Read the model definition and answer for the solid it produces. Units are mm, in the model's axes. A direction names the side the tool comes from. Give positions to 0.01 mm unless a question says otherwise; leave off trailing zeros. Write each loop counter-clockwise with the first axis right and the second up, starting at its lowest first coordinate (ties: lowest second). Pieces come first, ordered by that corner, then holes.
Autodesk Inventor part; units mm, degrees
ref_plane "YZ Plane" through (0, 0, 0) normal (1, 0, 0) x (0, 1, 0)
ref_plane "XZ Plane" through (0, 0, 0) normal (0, 1, 0) x (-1, 0, 0)
ref_plane "XY Plane" through (0, 0, 0) normal (0, 0, 1) x (1, 0, 0)
sketch "Sketch1" plane through (0, 0, 0) normal (1, 0, 0) x (0, 1, 0)
  line L0 (0, 0) -> (25.4, 0)
  line L1 (25.4, 0) -> (25.4, -25.4)
  line L2 (25.4, -25.4) -> (0, -25.4)
  line L3 (0, -25.4) -> (0, 0)
  dimension "d0" = 25.4
  dimension "d1" = 25.4
extrude "Extrusion1" add sketch "Sketch1" along normal blind 101.6
sketch "Sketch2" plane through (0, 0, 0) normal (-1, 0, 0) x (0, 0, 1)
  line L0 (-25.4, 0) -> (-25.4, 25.4)
  line L1 (-25.4, 0) -> (-21.59, 0)
  line L2 (-21.59, 3.81) -> (-17.78, 3.81)
  line L3 (-21.59, 7.62) -> (-21.59, 3.81)
  line L4 (-3.81, 21.59) -> (-7.62, 21.59)
  line L5 (-3.81, 17.78) -> (-3.81, 21.59)
  line L6 (-21.59, 3.81) -> (-3.81, 3.81)
  line L7 (-3.81, 3.81) -> (-3.81, 21.59)
  line L8 (-3.81, 21.59) -> (-21.59, 21.59)
  line L9 (-21.59, 21.59) -> (-21.59, 3.81)
  line L10 (-17.78, 7.62) -> (-7.62, 7.62)
  line L11 (-7.62, 7.62) -> (-7.62, 17.78)
  line L12 (-7.62, 17.78) -> (-17.78, 17.78)
  line L13 (-17.78, 17.78) -> (-17.78, 7.62)
  point P0 (0, 0)
  point P1 (0, 25.4)
extrude "Extrusion2" add sketch "Sketch2" along normal blind 38.1
sketch "Sketch3" plane through (101.6, 0, 0) normal (1, 0, 0) x (0, 0, -1)
  line L0 (0, 25.4) -> (0, 0)
  line L1 (25.4, 25.4) -> (0, 25.4)
  line L2 (3.302, 3.81) -> (3.302, 3.302)
  line L3 (3.302, 3.302) -> (3.81, 3.302)
  line L4 (3.302, 3.302) -> (22.098, 3.302)
  line L5 (22.098, 3.302) -> (22.098, 22.098)
  line L6 (22.098, 22.098) -> (3.302, 22.098)
  line L7 (3.302, 22.098) -> (3.302, 3.302)
  line L8 (8.128, 8.128) -> (17.272, 8.128)
  line L9 (17.272, 8.128) -> (17.272, 17.272)
  line L10 (17.272, 17.272) -> (8.128, 17.272)
  line L11 (8.128, 17.272) -> (8.128, 8.128)
  dimension "d32" = 0.508
  dimension "d33" = 0.508
extrude "Extrusion3" cut sketch "Sketch3" against normal blind 38.1
properties part number "Center Piece"
Item 1: Each of these flat-tipped pins is pushed along its axis until it touches: pin 1 Ø5.5 at (x, y) = (-12, 14) entering from -Z; pin 2 Ø5.5 at (x, z) = (-18.5, -14) entering from -Y; pin 3 Ø5 at (x, y) = (-13, 14.5) entering from +Z. Where does it stop, or does it pass through?
Result set:
pin 1: stops at z = -21.59
pin 2: stops at y = 3.81
pin 3: stops at z = -3.81
Item 2: Find the intervals of material crossed by line 1 along Z through (x, y) = (68.5, 13.75); line 2 along Y through (x, z) = (74, -11.75); line 3 along Z through (x, y) = (68, 19), in increasing order.
Result set:
line 1: z = -25.4 to -22.1, -17.27 to -8.13, -3.3 to 0
line 2: y = 0 to 3.3, 8.13 to 17.27, 22.1 to 25.4
line 3: z = -25.4 to -22.1, -3.3 to 0
Item 3: Section D-D (x = -19.5) is taken. Write down the section's boundary in (y, z).
Result set:
outline: (3.81, -21.59) - (21.59, -21.59) - (21.59, -3.81) - (3.81, -3.81) - close; hole (7.62, -17.78) - (17.78, -17.78) - (17.78, -7.62) - (7.62, -7.62) - close
Item 4: Determine the mould class of faces 5 (the flat face through (83, 13, -3.302)), 6 (the flat face through (-19, 13, -21.59)), 7 (the flat face through (-19, 7.62, -13)), 8 (the flat face through (101.6, 24, -13)) for opening direction Z: pulls with the +Z half, pulls with the -Z half, needs draft (parallel to the pull), parting line crosses it, or undercut.
Result set:
face 5: undercut
face 6: pulls with the -Z half
face 7: undercut
face 8: needs draft
Item 5: Which of the six approach directions +Z, -Z, +X, -X, +Y, -Y give full straight-line access (tool end or side, diameter ignored) to faces 1 (the flat face through (-19, 13, -7.62)), 2 (the flat face through (-19, 13, -3.81)), 3 (the flat face through (83, 13, -22.098)), 4 (the flat face through (-19, 21.59, -13))?
Result set:
face 1: -X
face 2: +Z, -X, +Y, -Y
face 3: +X
face 4: +Z, -Z, -X, +Y
Item 6: Section C-C (z = -14) is taken. Write down the section's boundary in (x, y), and give its area (3 significant figures).
Result set:
outline: (-38.1, 3.81) - (0, 3.81) - (0, 0) - (101.6, 0) - (101.6, 3.3) - (63.5, 3.3) - (63.5, 8.13) - (101.6, 8.13) - (101.6, 17.27) - (63.5, 17.27) - (63.5, 22.1) - (101.6, 22.1) - (101.6, 25.4) - (0, 25.4) - (0, 21.59) - (-38.1, 21.59) - (-38.1, 17.78) - (0, 17.78) - (0, 7.62) - (-38.1, 7.62) - close
area: 2,500 mm2
Item 7: Section A-A (x = 93.5) is taken. Write down the section's boundary in (y, z).
Result set:
outline: (0, -25.4) - (25.4, -25.4) - (25.4, 0) - (0, 0) - close; (8.13, -17.27) - (17.27, -17.27) - (17.27, -8.13) - (8.13, -8.13) - close; hole (3.3, -22.1) - (22.1, -22.1) - (22.1, -3.3) - (3.3, -3.3) - close
Item 8: Section B-B (y = 5.25) is taken. Write down the section's boundary in (x, z), and give its area (3 significant figures).
Result set:
outline: (-38.1, -21.59) - (0, -21.59) - (0, -25.4) - (101.6, -25.4) - (101.6, -22.1) - (63.5, -22.1) - (63.5, -3.3) - (101.6, -3.3) - (101.6, 0) - (0, 0) - (0, -3.81) - (-38.1, -3.81) - close
area: 2,540 mm2
